```python
from build123d import *

# Parameters (mm, degrees)
F0_W      = 366
F0_H      = 250
F1_DEPTH  = 155
F2_T      = -10
F3_W      = 346
F3_H      = 230
F4_DEPTH  = 25
F5_W      = 230
F5_H      = 15
F6_DEPTH  = 500
F7_W      = 240
F7_H      = 15
F8_DEPTH  = 500
F9_W      = 50
F9_H      = 10
F10_DEPTH = 366
F11_W     = 230
F11_H     = 6
F11_H_2   = 10
F12_DEPTH = 200
F13_W     = 22
F13_H     = 10
F14_DEPTH = 15
F15_W     = 22
F15_H     = 10
F16_DEPTH = 15
F17_DEPTH = 58
F18_DEPTH = 58
F19_DEPTH = 58
F20_DEPTH = 58
F21_R     = 5.5
F22_DEPTH = 235
F23_R     = 5.5
F24_DEPTH = 25
F25_R     = 5.5
F26_DEPTH = 240
F27_DEPTH = 260
F28_R     = 5.5
F29_DEPTH = 235
F30_R     = 5.5
F31_DEPTH = 5


with BuildPart() as f1:
    # F0 (on Top) → F1 (new body)
    with BuildSketch(Plane.XY):
        Rectangle(F0_W, F0_H)
    extrude(amount=F1_DEPTH)

    # F2
    f2_openings = [f1.faces().sort_by_distance(p)[0] for p in [
        (0, 0, 155),
    ]]
    offset(amount=F2_T, openings=f2_openings)

    # F3 (on face) → F4 (cut)
    with BuildSketch(Plane.XY.offset(10)):
        Rectangle(F3_W, F3_H)
    extrude(amount=-F4_DEPTH, mode=Mode.SUBTRACT)

    # F5 (on face) → F6 (cut)
    with BuildSketch(Plane.XZ.offset(125)):
        Polygon((115, 130), (-115, 130), (-115, 15), (0, 15), (115, 15), align=None)
        with Locations((0, 147.5)):
            Rectangle(F5_W, F5_H)
    extrude(amount=-F6_DEPTH, mode=Mode.SUBTRACT)

    # F7 (on face) → F8 (cut)
    with BuildSketch(Plane(origin=(-183, 0, 0), x_dir=(0, -1, 0), z_dir=(-1, 0, 0))):
        with Locations((-5, 147.5)):
            Rectangle(F7_W, F7_H)
        Polygon((-115, 15), (0, 15), (115, 15), (115, 130), (-115, 130), align=None)
    extrude(amount=-F8_DEPTH, mode=Mode.SUBTRACT)

    # F9 (on face) → F10 (join, through all)
    with BuildSketch(Plane(origin=(-183, 0, 0), x_dir=(0, -1, 0), z_dir=(-1, 0, 0))):
        with Locations((-140, 119)):
            Rectangle(F9_W, F9_H)
    extrude(amount=-F10_DEPTH)

    # F11 (on face) → F12 (cut)
    with BuildSketch(Plane(origin=(0, 125, 0), x_dir=(-1, 0, 0), z_dir=(0, 1, 0))):
        with Locations((0, 127)):
            Rectangle(F11_W, F11_H)
        with Locations((0, 135)):
            Rectangle(F11_W, F11_H_2)
    extrude(amount=-F12_DEPTH, mode=Mode.SUBTRACT)

    # F13 (on face) → F14 (join)
    with BuildSketch(Plane.XY.offset(140)):
        with Locations((126, 120)):
            Rectangle(F13_W, F13_H)
    extrude(amount=F14_DEPTH)

    # F15 (on face) → F16 (join)
    with BuildSketch(Plane.XY.offset(140)):
        with Locations((-126, 120)):
            Rectangle(F15_W, F15_H)
    extrude(amount=F16_DEPTH)

    # F17 (add, through all): a face of the model
    f17_faces = [f1.faces().sort_by_distance(p)[0] for p in [
        (173, 0, 135),
    ]]
    extrude(f17_faces, amount=F17_DEPTH)

    # F18 (add, through all): a face of the model
    f18_faces = [f1.faces().sort_by_distance(p)[0] for p in [
        (-173, 0, 135),
    ]]
    extrude(f18_faces, amount=F18_DEPTH)

    # F19 (add, through all): a face of the model
    f19_faces = [f1.faces().sort_by_distance(p)[0] for p in [
        (173, 0, 7.5),
    ]]
    extrude(f19_faces, amount=F19_DEPTH)

    # F20 (add, through all): a face of the model
    f20_faces = [f1.faces().sort_by_distance(p)[0] for p in [
        (-173, 0, 7.5),
    ]]
    extrude(f20_faces, amount=F20_DEPTH)

    # F21 (on face) → F22 (cut)
    with BuildSketch(Plane.XZ.offset(-115)):
        with Locations((125, 148)):
            Circle(F21_R)
    extrude(amount=F22_DEPTH, mode=Mode.SUBTRACT)

    # F23 (on face) → F24 (cut)
    with BuildSketch(Plane.XZ.offset(-115)):
        with Locations((-126, 148)):
            Circle(F23_R)
    extrude(amount=-F24_DEPTH, mode=Mode.SUBTRACT)

    # F25 (on face) → F26 (cut)
    with BuildSketch(Plane(origin=(115, 0, 0), x_dir=(0, -1, 0), z_dir=(-1, 0, 0))):
        with Locations((0, 7.5)):
            Circle(F25_R)
    extrude(amount=F26_DEPTH, mode=Mode.SUBTRACT)

    # F27 (cut): a face of the model
    f27_faces = [f1.faces().sort_by_distance(p)[0] for p in [
        (125, -120, 148),
    ]]
    extrude(f27_faces, amount=F27_DEPTH, mode=Mode.SUBTRACT)

    # F28 (on face) → F29 (cut)
    with BuildSketch(Plane.XZ.offset(-115)):
        with Locations((-126, 148)):
            Circle(F28_R)
    extrude(amount=F29_DEPTH, mode=Mode.SUBTRACT)

    # F30 (on face) → F31 (cut)
    with BuildSketch(Plane(origin=(115, 0, 0), x_dir=(0, -1, 0), z_dir=(-1, 0, 0))):
        with Locations((0, 7.5)):
            Circle(F30_R)
    extrude(amount=-F31_DEPTH, mode=Mode.SUBTRACT)


solid = f1.part
```
Work out the finished part from the listing and answer in its coordinate system (mm). A direction names the side the tool comes from. Round coordinates to 2 decimals unless told otherwise and drop trailing zeros. Loops run counter-clockwise (first coordinate to the right, second up) from the corner with the lowest first, then second, coordinate; pieces in that order, holes last.
(1) For faces 1 (the flat face through (120, 0, 8)), 2 (the flat face through (149, -115, 72)), 3 (the flat face through (-2, -115, 7)), 4 (the flat face through (-115, 120, 65)), determine the directions among +Z, -Z, +X, -X, +Y, -Y from which every point of the face is accessible in a straight line to the end or side of a thin tool.
Computed values:
face 1: none
face 2: +X, -X
face 3: +Z, -Z
face 4: +Y, -Y
(2) The part is cut by section C-C, the plane z = 148. Give the number of separate pieces and of enclosed holes in the cut face, and give its area (3 significant figures).
Computed values:
separate pieces: 6
enclosed holes: 0
area: 1,470 mm2
(3) The part is cut by section A-A, the plane y = 96. Give the vertices of the cut face in (x, z).
Computed values:
outline: (-183, 0) - (-115, 0) - (-115, 15) - (-183, 15) - close; (-183, 130) - (-115, 130) - (-115, 140) - (-183, 140) - close; (115, 0) - (183, 0) - (183, 15) - (115, 15) - close; (115, 130) - (183, 130) - (183, 140) - (115, 140) - close
(4) Each of these flat-tipped pins is pushed along its axis until it touches: P1, Ø20.5, axis at x = -154.5, y = 36.5, coming from the +Z side; P2, Ø25, axis at x = -159, z = 139, coming from the +Y side; P3, Ø3, axis at y = 120, z = 150, coming from the -X side. Where does it stop, or does it pass through?
Computed values:
P1: stops at z = 140
P2: stops at y = 125
P3: stops at x = -137
(5) Find the intervals of material crossed by L1, parallel to Z at x = -122.5, y = 0; L2, parallel to Y at x = 117, z = 72; L3, parallel to Z at x = -126, y = -118.9, in increasing order.
Computed values:
L1: z = 0 to 2, 13 to 15, 130 to 140
L2: y = -125 to -115, 115 to 125
L3: z = 0 to 142.5, 153.5 to 155
(6) The part is cut by section B-B, the plane x = 125. Give the vertices of the cut face in (y, z).
Computed values:
outline: (-125, 0) - (125, 0) - (125, 114) - (165, 114) - (165, 124) - (125, 124) - (125, 142.5) - (115, 142.5) - (115, 140) - (-115, 140) - (-115, 142.5) - (-120, 142.5) - (-120, 153.5) - (-115, 153.5) - (-115, 155) - (-125, 155) - close; (115, 153.5) - (125, 153.5) - (125, 155) - (115, 155) - close; hole (-115, 15) - (115, 15) - (115, 130) - (-115, 130) - close
(7) The part is cut by section D-D, the plane x = -87.5. Give the vertices of the cut face in (y, z).
Computed values:
outline: (-125, 0) - (-115, 0) - (-115, 15) - (-125, 15) - close; (-125, 130) - (-115, 130) - (-115, 140) - (-125, 140) - close; (115, 0) - (125, 0) - (125, 15) - (115, 15) - close; (115, 114) - (165, 114) - (165, 124) - (115, 124) - close
(8) The mould has two halves that part along X. Classify faces 5 (the flat face through (-115, 13, 136)), 6 (the flat face through (-2, -115, 135)), 7 (the flat face through (-3, -125, 8)), 8 (the flat face through (-183, 9.9, 14.7)): pulls with the +X half, pulls with the -X half, needs draft (parallel to the pull), parting line crosses it, or undercut.
Computed values:
face 5: undercut
face 6: undercut
face 7: needs draft
face 8: pulls with the -X half
